Input: part model. Units: mm. Frame: model coordinates. Coordinates: 2 decimals unless noted, no trailing zeros. Write each loop counter-clockwise with the first axis right and the second up, starting at its lowest first coordinate (ties: lowest second). Pieces come first, ordered by that corner, then holes. Notation, with made-up numbers: (17.5, -21) - (45.5, -21) arc R11 ccw to (45.5, -5) - close; hole circle Ø3 at (46.5, 78.25). An arc over 180 degrees is marked (long way). Use CSV: the item, a comma, the result in double quotes.
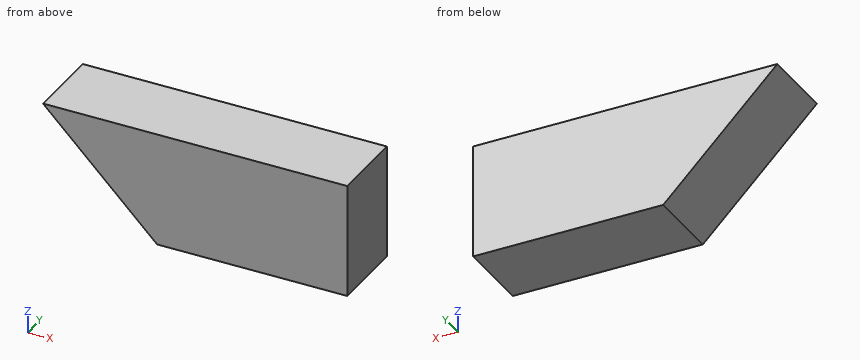
```python
from build123d import *

# Parameters (mm, degrees)
F0_W     = 8
F0_H     = 2
F1_DEPTH = 3
F2_SIZE  = 2.99999


# Not quite as in the source:
# - a fillet or chamfer is up to 0.001 mm smaller than in the source, because OpenCascade refuses the exact size


with BuildPart() as f1:
    # F0 (on Top) → F1 (new body)
    with BuildSketch(Plane.XY):
        Rectangle(F0_W, F0_H)
    extrude(amount=F1_DEPTH)

    # F2 (size 3 in the source; OpenCascade refuses exactly that, so slightly less here)
    f2_edges = [f1.edges().sort_by_distance(p)[0] for p in [
        (-4, 0, 0),
    ]]
    chamfer(f2_edges, length=F2_SIZE)


solid = f1.part
```
(1) Cut plane B-B on z = 1.45. Return loops of the section in (x, y).
Check values:
outline,"(-2.45, -1) - (4, -1) - (4, 1) - (-2.45, 1) - close"
(2) Ray query, probe 1 along X at (y, z) = (-0.65, 2.3); probe 2 along X at (y, z) = (-0.1, 1.15); probe 3 along Z at (x, y) = (-3, 0.5). Return the intervals inside material, ascending. Write a range as from..to.
Check values:
probe 1,"-3.3..4"
probe 2,"-2.15..4"
probe 3,"2..3"
(3) Cut plane C-C on x = -3.5. Return loops of the section in (y, z).
Check values:
outline,"(-1, 2.5) - (1, 2.5) - (1, 3) - (-1, 3) - close"
